Source: CAD feature listing. Evaluate the final solid. Frame: model axes, mm. Face numbers are marked on the shaded views. A direction names the side the tool comes from. Give positions to 0.01 mm unless a question says otherwise; leave off trailing zeros. Write each loop counter-clockwise with the first axis right and the second up, starting at its lowest first coordinate (ties: lowest second). Pieces come first, ordered by that corner, then holes. Notation, with made-up numbers: M 13.25,1 L 56.25,1 A34 cw 56.25,37 Z; hole C -27,54 d7. An arc over 180 degrees is marked long. Return JSON: item names as keys, results as strings.
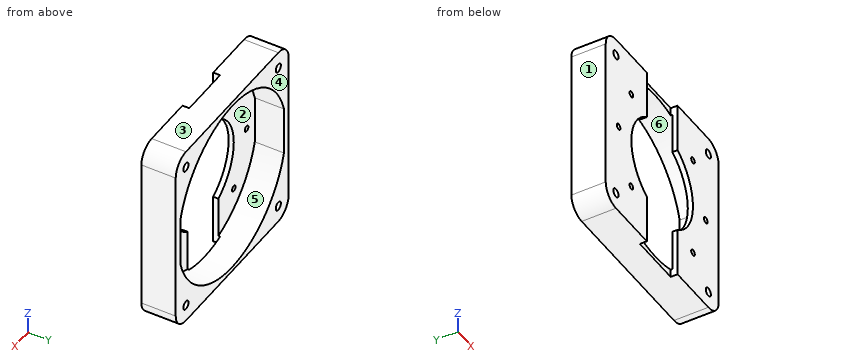
```python
from build123d import *

# Parameters (mm, degrees)
SKETCH_1_W          = 110
SKETCH_1_H          = 110
EXTRUDE_5_DEPTH     = 20
CUT_EXTRUDE_2_DEPTH = 17
SKETCH_5_R          = 1.75
SKETCH_5_R_2        = 30
CUT_EXTRUDE_3_DEPTH = 17
SKETCH_7_W          = 30
SKETCH_7_H          = 114.29986349
CUT_EXTRUDE_4_DEPTH = 4
SKETCH_8_R          = 2.5
CUT_EXTRUDE_5_DEPTH = 81.311892021
FILLET_1_R          = 10
FILLET_2_R          = 10
FILLET_3_R          = 10
FILLET_4_R          = 10
CUT_EXTRUDE_6_DEPTH = 17
CUT_EXTRUDE_7_DEPTH = 17


with BuildPart() as part:
    # 草图1 → 凸台-拉伸5 (new body)
    with BuildSketch(Plane(origin=(0, 0, 0), x_dir=(1, 0, 0), z_dir=(0, 1, 0))):
        Rectangle(SKETCH_1_W, SKETCH_1_H)
    extrude(amount=EXTRUDE_5_DEPTH)

    # 草图4 → 切除-拉伸2 (cut)
    with BuildSketch(Plane(origin=(0, 20, 0), x_dir=(1, 0, 0), z_dir=(0, 1, 0))):
        with BuildLine():
            ThreePointArc((-47, -13.856406461), (0, -49), (47, -13.856406461))
            Line((47, -13.856406461), (47, 13.856406461))
            ThreePointArc((47, 13.856406461), (0, 49), (-47, 13.856406461))
            Line((-47, 13.856406461), (-47, -13.856406461))
        make_face()
    extrude(amount=-CUT_EXTRUDE_2_DEPTH, mode=Mode.SUBTRACT)

    # 草图5 → 切除-拉伸3 (cut)
    with BuildSketch(Plane(origin=(0, 3, 0), x_dir=(1, 0, 0), z_dir=(0, 1, 0))):
        with Locations(Location((0, 42.5, 0), (0, 0, 270))):
            Circle(SKETCH_5_R)
        with Locations(Location((30.0520382, 30.0520382, 0), (0, 0, 270))):
            Circle(SKETCH_5_R)
        with Locations(Location((42.5, 0, 0), (0, 0, 270))):
            Circle(SKETCH_5_R)
        with Locations(Location((30.0520382, -30.0520382, 0), (0, 0, 270))):
            Circle(SKETCH_5_R)
        with Locations(Location((0, -42.5, 0), (0, 0, 270))):
            Circle(SKETCH_5_R)
        with Locations(Location((-30.0520382, -30.0520382, 0), (0, 0, 270))):
            Circle(SKETCH_5_R)
        with Locations(Location((-42.5, 0, 0), (0, 0, 270))):
            Circle(SKETCH_5_R)
        with Locations(Location((-30.0520382, 30.0520382, 0), (0, 0, 270))):
            Circle(SKETCH_5_R)
        with Locations(Location((0, 0, 0), (0, 0, 270))):
            Circle(SKETCH_5_R_2)
    extrude(amount=-CUT_EXTRUDE_3_DEPTH, mode=Mode.SUBTRACT)

    # 草图7 → 切除-拉伸4 (cut)
    with BuildSketch(Plane.XZ):
        Rectangle(SKETCH_7_W, SKETCH_7_H)
    extrude(amount=-CUT_EXTRUDE_4_DEPTH, mode=Mode.SUBTRACT)

    # 草图8 → 切除-拉伸5 (cut, through all)
    with BuildSketch(Plane(origin=(0, 20, 0), x_dir=(1, 0, 0), z_dir=(0, 1, 0))):
        with Locations(Location((45, 45, 0), (0, 0, 270))):
            Circle(SKETCH_8_R)
        with Locations(Location((45, -45, 0), (0, 0, 270))):
            Circle(SKETCH_8_R)
        with Locations(Location((-45, -45, 0), (0, 0, 270))):
            Circle(SKETCH_8_R)
        with Locations(Location((-45, 45, 0), (0, 0, 270))):
            Circle(SKETCH_8_R)
    extrude(amount=-CUT_EXTRUDE_5_DEPTH, mode=Mode.SUBTRACT)

    # 圆角1
    fillet_1_edges = [part.edges().sort_by_distance(p)[0] for p in [
        (55, 10, -55),
    ]]
    fillet(fillet_1_edges, radius=FILLET_1_R)

    # 圆角2
    fillet_2_edges = [part.edges().sort_by_distance(p)[0] for p in [
        (-55, 10, -55),
    ]]
    fillet(fillet_2_edges, radius=FILLET_2_R)

    # 圆角3
    fillet_3_edges = [part.edges().sort_by_distance(p)[0] for p in [
        (-55, 10, 55),
    ]]
    fillet(fillet_3_edges, radius=FILLET_3_R)

    # 圆角4
    fillet_4_edges = [part.edges().sort_by_distance(p)[0] for p in [
        (55, 10, 55),
    ]]
    fillet(fillet_4_edges, radius=FILLET_4_R)

    # 草图10 → 切除-拉伸6 (cut)
    with BuildSketch(Plane(origin=(0, 20, 0), x_dir=(1, 0, 0), z_dir=(0, 1, 0))):
        with BuildLine():
            Line((50, -14.282856857), (50, 14.282856857))
            ThreePointArc((50, 14.282856857), (0, 52), (-50, 14.282856857))
            Line((-50, 14.282856857), (-50, -14.282856857))
            ThreePointArc((-50, -14.282856857), (0, -52), (50, -14.282856857))
        make_face()
    extrude(amount=-CUT_EXTRUDE_6_DEPTH, mode=Mode.SUBTRACT)

    # 草图11 → 切除-拉伸7 (cut)
    with BuildSketch(Plane(origin=(0, 20, 0), x_dir=(1, 0, 0), z_dir=(0, 1, 0))):
        with BuildLine():
            Line((50.5, -14.352700094), (50.5, 14.352700094))
            ThreePointArc((50.5, 14.352700094), (0, 52.5), (-50.5, 14.352700094))
            Line((-50.5, 14.352700094), (-50.5, -14.352700094))
            ThreePointArc((-50.5, -14.352700094), (0, -52.5), (50.5, -14.352700094))
        make_face()
    extrude(amount=-CUT_EXTRUDE_7_DEPTH, mode=Mode.SUBTRACT)


solid = part.part
```
1) Cut plane B-B, the plane y = 17.5. Return the cut outline in (x, z).
Numbers:
{"outline": "M -55,-45 A10 ccw -45,-55 L 45,-55 A10 ccw 55,-45 L 55,45 A10 ccw 45,55 L -45,55 A10 ccw -55,45 Z; hole M -50.5,-14.35 A52.5 ccw 50.5,-14.35 L 50.5,14.35 A52.5 ccw -50.5,14.35 Z; hole C -45,-45 d5; hole C -45,45 d5; hole C 45,-45 d5; hole C 45,45 d5"}
2) Line query: line 1 (Z direction, x = 1.5, y = 18.75); line 2 (Z direction, x = 46, y = 5.75); line 3 (X direction, y = 9, z = 10.5). Output: solid intervals per line, ascending. Write a range as [from, to].
Numbers:
{"line 1": "z = [-55, -52.48], [52.48, 55]", "line 2": "z = [-54.95, -47.29], [-42.71, -25.3], [25.3, 42.71], [47.29, 54.95]", "line 3": "x = [-55, -50.5], [50.5, 55]"}
3) Set-up query: the marked faces 1 and 2. Return all of +Z, -Z, +X, -X, +Y, -Y with unobstructed straight access to the full face (end or side cutting, diameter ignored); none if empty.
Numbers:
{"face 1": "+Z, -Z, -X, +Y, -Y", "face 2": "+Y"}
4) Draft query along Z for the marked faces 3, 4, 5 and 6. Return one class per face: released by +Z, released by -Z, zero draft, split by the parting line, or undercut.
Numbers:
{"face 3": "released by +Z", "face 4": "zero draft", "face 5": "undercut", "face 6": "undercut"}
5) Cut plane C-C, the plane x = 9.5. Return the cut outline in (y, z), then the cut area to 3 significant figures.
Numbers:
{"outline": "M 4,-55 L 20,-55 L 20,-51.63 L 4,-51.63 Z; M 4,51.63 L 20,51.63 L 20,55 L 4,55 Z", "area": "108 mm²"}
6) Cut plane A-A, the plane z = 0. Return the cut outline in (x, y).
Numbers:
{"outline": "M -55,0 L -44.25,0 L -44.25,3 L -50.5,3 L -50.5,20 L -55,20 Z; M -40.75,0 L -30,0 L -30,3 L -40.75,3 Z; M 30,0 L 40.75,0 L 40.75,3 L 30,3 Z; M 44.25,0 L 55,0 L 55,20 L 50.5,20 L 50.5,3 L 44.25,3 Z"}
7) Contact query for flat-ended pins moving along their axis: pin 1 Ø18 at (x, z) = (-29.5, -20) entering from +Y; pin 2 Ø3 at (y, z) = (2.5, 47) entering from -X; pin 3 Ø4 at (x, z) = (-5.5, -52.5) entering from -Y. Output: stop coordinate, or through.
Numbers:
{"pin 1": "stops at y = 3", "pin 2": "stops at x = -54.99", "pin 3": "stops at y = 4"}
